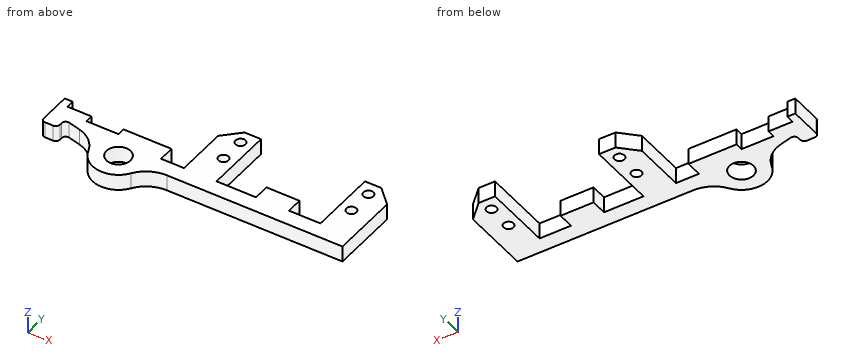
```python
from build123d import *

# Parameters (mm, degrees)
SKETCH1_W               = 12.9
SKETCH1_H               = 6.35
BOSS_EXTRUDE1_DEPTH     = 6.35
BOSS_EXTRUDE1_2_DEPTH   = 6.35
SKETCH1_W_2             = 13.1
BOSS_EXTRUDE1_3_DEPTH   = 6.35
BOSS_EXTRUDE1_4_DEPTH   = 6.35
SKETCH2_W               = 88.9
SKETCH2_H               = 6.35
BOSS_EXTRUDE2_DEPTH     = 12.7
SKETCH3_W               = 12.9
SKETCH3_H               = 6.35
BOSS_EXTRUDE3_DEPTH     = 20.6375
CHAMFER1_SIZE           = 6.35
SKETCH4_R               = 1.984375
CUT_EXTRUDE1_DEPTH      = 7.35
SKETCH12_W              = 6.35
SKETCH12_H              = 12.7
BOSS_EXTRUDE6_DEPTH     = 0.2
SKETCH13_W              = 89.1
SKETCH13_H              = 6.35
CUT_EXTRUDE2_DEPTH      = 7.35
BOSS_EXTRUDE7_DEPTH     = 6.35
SKETCH19_R              = 10.31875
SKETCH19_R_2            = 4.7625
BOSS_EXTRUDE8_DEPTH     = 6.35
SKETCH20_R              = 4.7625
CUT_EXTRUDE3_DEPTH      = 1
CUT_EXTRUDE3_DEPTH_BACK = 7.35
FILLET2_R               = 12.7
SKETCH21_W              = 6.35
SKETCH21_H              = 6.35
BOSS_EXTRUDE9_DEPTH     = 6.35
FILLET4_R               = 1.5875
SKETCH22_W              = 12.7
SKETCH22_H              = 3.048
CUT_EXTRUDE4_DEPTH      = 7.35


with BuildPart() as part:
    # Sketch1 → Boss-Extrude1 (new body)
    with BuildSketch(Plane(origin=(0, 136.676286052, 0), x_dir=(1, 0, 0), z_dir=(0, 1, 0))):
        with Locations((-97.400963438, -57.278255958)):
            Rectangle(SKETCH1_W, SKETCH1_H)
    extrude(amount=-BOSS_EXTRUDE1_DEPTH)



with BuildPart() as body_2:
    # Sketch1 → Boss-Extrude1 2 (new body)
    with BuildSketch(Plane(origin=(0, 136.676286052, 0), x_dir=(1, 0, 0), z_dir=(0, 1, 0))):
        with Locations((-75.375963438, -57.278255958)):
            Rectangle(SKETCH1_W, SKETCH1_H)
    extrude(amount=-BOSS_EXTRUDE1_2_DEPTH)


with BuildPart() as body_3:
    # Sketch1 → Boss-Extrude1 3 (new body)
    with BuildSketch(Plane(origin=(0, 136.676286052, 0), x_dir=(1, 0, 0), z_dir=(0, 1, 0))):
        with Locations((-46.700963438, -57.278255958)):
            Rectangle(SKETCH1_W_2, SKETCH1_H)
    extrude(amount=-BOSS_EXTRUDE1_3_DEPTH)


with BuildPart() as body_4:
    # Sketch1 → Boss-Extrude1 4 (new body)
    with BuildSketch(Plane(origin=(0, 136.676286052, 0), x_dir=(1, 0, 0), z_dir=(0, 1, 0))):
        with Locations((-21.200963438, -57.278255958)):
            Rectangle(SKETCH1_W, SKETCH1_H)
    extrude(amount=-BOSS_EXTRUDE1_4_DEPTH)


with BuildPart() as part_1:
    add(part.part)

    add(body_2.part)  # Boss-Extrude2 merges body 2

    add(body_3.part)  # Boss-Extrude2 merges body 3

    add(body_4.part)  # Boss-Extrude2 merges body 4
    # Sketch2 → Boss-Extrude2 (add)
    with BuildSketch(Plane(origin=(0, 130.326286052, 0), x_dir=(-1, 0, 0), z_dir=(0, -1, 0))):
        with Locations((59.400963438, -57.278255958)):
            Rectangle(SKETCH2_W, SKETCH2_H)
    extrude(amount=BOSS_EXTRUDE2_DEPTH)

    # Sketch3 → Boss-Extrude3 (add)
    with BuildSketch(Plane(origin=(0, 136.676286052, 0), x_dir=(1, 0, 0), z_dir=(0, 1, 0))):
        with Locations((-75.375963438, -57.278255958)):
            Rectangle(SKETCH3_W, SKETCH3_H)
        with Locations((-21.200963438, -57.278255958)):
            Rectangle(SKETCH3_W, SKETCH3_H)
    extrude(amount=BOSS_EXTRUDE3_DEPTH)

    # Chamfer1
    chamfer1_edges = [part_1.edges().sort_by_distance(p)[0] for p in [
        (-81.825963438, 157.313786052, 57.278255958),
        (-14.750963438, 157.313786052, 57.278255958),
    ]]
    chamfer(chamfer1_edges, length=CHAMFER1_SIZE)

    # Sketch4 → Cut-Extrude1 (cut, through all)
    with BuildSketch(Plane.XY.offset(60.453255958)):
        with Locations((-73.688463438, 152.154411052)):
            Circle(SKETCH4_R)
        with Locations((-73.688463438, 141.835661052)):
            Circle(SKETCH4_R)
        with Locations((-22.888463438, 141.835661052)):
            Circle(SKETCH4_R)
        with Locations((-22.888463438, 152.154411052)):
            Circle(SKETCH4_R)
    extrude(amount=-CUT_EXTRUDE1_DEPTH, mode=Mode.SUBTRACT)

    # Sketch12 → Boss-Extrude6 (add)
    with BuildSketch(Plane(origin=(-14.950963438, 0, 0), x_dir=(0, 0, -1), z_dir=(1, 0, 0))):
        with Locations((-57.278255958, 123.976286052)):
            Rectangle(SKETCH12_W, SKETCH12_H)
    extrude(amount=BOSS_EXTRUDE6_DEPTH)

    # Sketch13 → Cut-Extrude2 (cut, through all)
    with BuildSketch(Plane.XY.offset(60.453255958)):
        with Locations((-59.300963438, 120.801286052)):
            Rectangle(SKETCH13_W, SKETCH13_H)
    extrude(amount=-CUT_EXTRUDE2_DEPTH, mode=Mode.SUBTRACT)

    # Sketch14 → Boss-Extrude7 (add)
    with BuildSketch(Plane.XY.offset(60.453255958)):
        Polygon((-132.250963468, 139.851286052), (-135.425963468, 139.851286052), (-135.425963468, 131.913786052), (-103.850963438, 123.976286052), (-103.850963438, 136.676286052), (-132.250963468, 136.676286052), align=None)
    extrude(amount=-BOSS_EXTRUDE7_DEPTH)

    # Sketch19 → Boss-Extrude8 (add)
    with BuildSketch(Plane.XY.offset(60.453255958)):
        with Locations((-103.675963468, 123.976286052)):
            Circle(SKETCH19_R)
        with Locations((-103.675963468, 123.976286052)):
            Circle(SKETCH19_R_2, mode=Mode.SUBTRACT)
    extrude(amount=-BOSS_EXTRUDE8_DEPTH)

    # Sketch20 → Cut-Extrude3 (cut, two sides)
    with BuildSketch(Plane.XY.offset(60.453255958)) as cut_extrude3_sk:
        with Locations((-103.675963468, 123.976286052)):
            Circle(SKETCH20_R)
    extrude(amount=CUT_EXTRUDE3_DEPTH, mode=Mode.SUBTRACT)
    extrude(cut_extrude3_sk.sketch, amount=-CUT_EXTRUDE3_DEPTH_BACK, mode=Mode.SUBTRACT)

    # Fillet2
    fillet2_edges = [part_1.edges().sort_by_distance(p)[0] for p in [
        (-113.693666461, 126.450599755, 57.278255958),
        (-93.357213468, 123.976286052, 57.278255958),
    ]]
    fillet(fillet2_edges, radius=FILLET2_R)

    # Sketch21 → Boss-Extrude9 (add)
    with BuildSketch(Plane.XY.offset(60.453255958)):
        with Locations((-132.250963468, 128.738786052)):
            Rectangle(SKETCH21_W, SKETCH21_H)
    extrude(amount=-BOSS_EXTRUDE9_DEPTH)

    # Fillet4
    fillet4_edges = [part_1.edges().sort_by_distance(p)[0] for p in [
        (-129.075963468, 130.317487558, 57.278255958),
        (-129.075963468, 125.563786052, 57.278255958),
        (-135.425963468, 125.563786052, 57.278255958),
    ]]
    fillet(fillet4_edges, radius=FILLET4_R)

    # Sketch22 → Cut-Extrude4 (cut, through all)
    with BuildSketch(Plane.XY.offset(60.453255958)):
        with Locations((-116.350963438, 135.152286052)):
            Rectangle(SKETCH22_W, SKETCH22_H)
    extrude(amount=-CUT_EXTRUDE4_DEPTH, mode=Mode.SUBTRACT)


solid = part_1.part
```
Input: part model. Units: mm. Frame: model coordinates. Coordinates: 2 decimals unless noted, no trailing zeros. Loops run counter-clockwise (first coordinate to the right, second up) from the corner with the lowest first, then second, coordinate; pieces in that order, holes last. Notation, with made-up numbers: M 8.25,28.5 L 47.25,28.5 A14 ccw 47.25,54.5 Z; hole C -1,66 d9. An arc over 180 degrees is marked long. Use a Markdown table: item, result. Add a question column.
1) Section A-A, the plane y = 148. Return the cut outline in (x, z).
2) Section B-B, the plane x = -51.5. Return the cut outline in (y, z).
3) Section D-D, the plane y = 117. Return the cut outline in (x, z).
4) Pin query (flat end, axial travel): P1, Ø2, axis at x = -108.5, z = 59, coming from the +Y side; P2, Ø3, axis at x = -30.5, z = 56.5, coming from the -Y side; P3, Ø1, axis at y = 152.5, z = 59, coming from the -X side. Return the tip coordinate at first contact, or that it passes through.
5) Section C-C, the plane z = 57. Give the number of separate pieces and of enclosed holes in the cut face, plus the area to 3 significant figures.
6) Line query: L1, parallel to X at y = 139, z = 58; L2, parallel to X at y = 132.5, z = 56.5; L3, parallel to X at y = 146.5, z = 58. Output: solid intervals per line, ascending. Write a range as from..to.
Answer below:
| question | item | result |
|---|---|---|
| 1 | outline | M -81.83,54.1 L -68.93,54.1 L -68.93,60.45 L -81.83,60.45 Z; M -27.65,54.1 L -14.75,54.1 L -14.75,60.45 L -27.65,60.45 Z |
| 2 | outline | M 123.98,54.1 L 136.68,54.1 L 136.68,60.45 L 123.98,60.45 Z |
| 3 | outline | M -111.28,54.1 L -96.07,54.1 L -96.07,60.45 L -111.28,60.45 Z |
| 4 | P1 | y = 136.68 |
| 4 | P2 | y = 123.98 |
| 4 | P3 | x = -80.79 |
| 5 | separate pieces | 1 |
| 5 | enclosed holes | 5 |
| 5 | area | 1,750 mm2 |
| 6 | L1 | -135.43..-132.25, -81.83..-68.93, -27.65..-14.75 |
| 6 | L2 | -135.43..-90.95, -81.83..-68.93, -53.25..-40.15, -27.65..-14.75 |
| 6 | L3 | -81.83..-68.93, -27.65..-14.75 |
